Autodesk Inventor part; units mm, degrees
ref_plane "YZ Plane" through (0, 0, 0) normal (1, 0, 0) x (0, 1, 0)
ref_plane "XZ Plane" through (0, 0, 0) normal (0, 1, 0) x (-1, 0, 0)
ref_plane "XY Plane" through (0, 0, 0) normal (0, 0, 1) x (1, 0, 0)
sketch "Sketch1" plane through (0, 0, 0) normal (0, 1, 0) x (-1, 0, 0)
  circle A0 centre (-7.6905, 26.7159) radius 1.5
  circle A1 centre (-7.6905, 14.7159) radius 1.5
  line L0 (-0.1905, 5.7159) -> (-15.1905, 5.7159)
  line L1 (-15.1905, 35.7159) -> (-0.1905, 35.7159)
  line L2 (-15.1905, 5.7159) -> (-15.1905, 35.7159)
  circle A2 centre (5.6845, 41.7159) radius 1.5
  circle A3 centre (5.6845, 41.7159) radius 2.75
  line L3 (-2.528, 47.7159) -> (7.472, 47.7159)
  circle A4 centre (50.4345, -18.1591) radius 2.75
  circle A5 centre (50.4345, -36.2841) radius 1.5
  line L4 (9.8095, -42.2841) -> (9.8095, -22.2841)
  circle A6 centre (50.4345, -18.1591) radius 1.5
  line L5 (-0.1905, 35.7159) -> (-0.1905, 5.7159)
  line L6 (56.4345, 47.7159) -> (7.472, 47.7159)
  circle A7 centre (50.4345, 23.5909) radius 1.5
  line L7 (56.4345, -42.2841) -> (56.4345, 47.7159)
  line L8 (42.1595, 2.7159) -> (61.2095, 2.7159) construction
  circle A8 centre (50.4345, 23.5909) radius 2.75
  line L9 (-15.1905, 35.7159) -> (-30.1905, 35.7159)
  line L10 (-63.5655, 30.7159) -> (-63.5655, 47.7159)
  line L11 (-63.5655, 47.7159) -> (-48.5655, 47.7159)
  line L12 (-2.528, 47.7159) -> (-63.5655, 47.7159)
  circle A9 centre (-36.0655, 41.7159) radius 1.5
  circle A10 centre (-36.0655, 41.7159) radius 2.75
  circle A11 centre (-21.1905, -7.2841) radius 1.5
  line L13 (-27.6905, 2.7159) -> (-27.6905, -17.2841)
  circle A12 centre (-57.5655, -34.7841) radius 1.5
  line L14 (-2.6905, 2.7159) -> (-27.6905, 2.7159)
  circle A13 centre (-9.1905, -7.2841) radius 1.5
  line L15 (-2.6905, -17.2841) -> (-2.6905, 2.7159)
  line L16 (-27.6905, -17.2841) -> (-2.6905, -17.2841)
  line L17 (-63.5655, 47.7159) -> (-63.5655, -42.2841)
  line L18 (9.8095, -22.2841) -> (-40.1905, -22.2841)
  line L19 (-40.1905, -22.2841) -> (-40.1905, -42.2841)
  line L20 (-40.1905, -42.2841) -> (9.8095, -42.2841)
  line L21 (-63.5655, -42.2841) -> (56.4345, -42.2841)
  line L22 (-63.5655, 28.0659) -> (-48.5655, 28.0659)
  circle A14 centre (-22.6905, 26.7159) radius 1.5
  circle A15 centre (-53.0655, 20.5659) radius 1.5
  circle A16 centre (-59.0655, 20.5659) radius 1.5
  circle A17 centre (-53.0655, 20.5659) radius 2.5
  circle A18 centre (-22.6905, 14.7159) radius 1.5
  line L23 (-15.1905, 5.7159) -> (-15.1905, 35.7159)
  line L24 (-30.1905, 5.7159) -> (-15.1905, 5.7159)
  line L25 (-48.5655, 28.0659) -> (-48.5655, 13.0659)
  line L26 (-30.1905, 35.7159) -> (-30.1905, 5.7159)
  circle A19 centre (-59.0655, 20.5659) radius 2.5
  line L27 (-48.5655, 13.0659) -> (-63.5655, 13.0659)
  line L28 (-63.5655, 13.0659) -> (-63.5655, 28.0659)
  line L29 (-15.1905, 2.7159) -> (-15.1905, 34.925) construction
  line L30 (-48.5655, 28.0659) -> (-40.5655, 28.0659)
  line L31 (-40.5655, 28.0659) -> (-40.5655, 47.7159)
  point P0 (0, 0)
  point P1 (5.1035, 21.0043)
  point P2 (5.6845, 35.7159)
  point P3 (2.472, 2.7159)
  point P4 (-36.0655, 35.7159)
  point P5 (-2.6905, -7.2841)
  point P6 (-43.5655, 47.7159)
  dimension "d4" = 12
  dimension "d5" = 7.5
  dimension "d6" = 12
  dimension "d7" = 9
  dimension "d8" = 0
  dimension "d10" = 0
  dimension "d12" = 8
  dimension "d13" = 5.5
  dimension "d14" = 5.5
  dimension "d15" = 5.5
  dimension "d16" = 5.5
extrude "Extrusion1" add sketch "Sketch1" along normal blind 4 contours L3 L6 L7 L21 L4 L18 L19 L17 L27 L25 L30 L31 L12
extrude "Extrusion2" add sketch "Sketch1" along normal blind 2 contours L0 L2 L1 L5 | L24 L26 L9 L2 | A3 | L25 L27 L17 L22 | A4 | A8 | A10 | L14 L15 L16 L13 | A17 | A19
properties part number "Casis Kanan Bawah_3DPrint"
Build history of the part. All positions in model axes, mm. A direction names the side the tool comes from. Give positions to 0.01 mm unless a question says otherwise; leave off trailing zeros. Order: outer loops, then holes, each group sorted by start corner. A loop starts at its lowest first (then second) coordinate and runs counter-clockwise, first axis right, second up. Notation, with made-up numbers: M 50.25,-26 L 103.25,-26 A13 ccw 103.25,-5 Z; hole C 27.5,3.5 d1. An arc over 180 degrees is marked long. Put each result on its own line as item: value.
Item 1: Slice it at A-A, the plane z = -26. Write the cut outline in (x, y).
From the geometry:
outline: M -56.43,0 L -9.81,0 L -9.81,4 L -56.43,4 Z; M 40.19,0 L 63.57,0 L 63.57,4 L 40.19,4 Z
Item 2: Slice it at B-B, the plane z = 32. Write the cut outline in (x, y).
From the geometry:
outline: M -56.43,0 L 40.57,0 L 40.57,4 L 30.19,4 L 30.19,2 L 0.19,2 L 0.19,4 L -56.43,4 Z
Item 3: 3-axis set-ups, long thin cutter, end or side, ignore diameter. For faces 5 (the flat face through (15, 2, 21)), 6 (the flat face through (56, 2, 21)), 7 (the cylindrical face through (-51.127, 1.972, -34.953)): which of +Z, -Z, +X, -X, +Y, -Y reach the whole face in a straight line?
From the geometry:
face 5: +Y
face 6: +Z, +X, +Y
face 7: +Y, -Y
Item 4: Slice it at D-D, the plane x = 17.5. Write the cut outline in (y, z), plus the area to 3 significant figures.
From the geometry:
outline: M 0,-22.28 L 4,-22.28 L 4,-17.28 L 2,-17.28 L 2,2.72 L 4,2.72 L 4,5.72 L 2,5.72 L 2,35.72 L 4,35.72 L 4,47.72 L 0,47.72 Z
area: 180 mm2
Item 5: Probe line 1 (Z direction, x = 11, y = 3.1); line 2 (X direction, y = 3.85, z = -27); line 3 (Z direction, x = 21, y = 1.3). List the from-to ranges inside material, lowest first. Write a range as [from, to].
From the geometry:
line 1: z = [-22.28, -17.28], [2.72, 5.72], [35.72, 47.72]
line 2: x = [-56.43, -9.81], [40.19, 63.57]
line 3: z = [-22.28, -8.77], [-5.8, 47.72]
Item 6: Slice it at C-C, the plane y = 3.4. Give the number of separate pieces and of enclosed holes in the cut face, plus the area to 3 significant figures.
From the geometry:
separate pieces: 1
enclosed holes: 8
area: 7,610 mm2
Item 7: Flat gauge pins, fed straight in: pin 1 Ø6 at (x, z) = (37, 41) entering from +Y; pin 2 Ø2.5 at (x, z) = (-50.43, -18.16) entering from +Y; pin 3 Ø3.5 at (x, z) = (22.69, 26.72) entering from +Y; pin 4 Ø0.6 at (y, z) = (3, 24) entering from +X. Where does each tip first touch, or does it go through?
From the geometry:
pin 1: stops at y = 4
pin 2: passes through
pin 3: stops at y = 2
pin 4: stops at x = 48.57
Item 8: Two-plate mould, pull along Z, no slides. Class faces 1 (the flat face through (-56.434, 2, 2)), 2 (the flat face through (49.7, 1.5, 28.066)), 3 (the cylindrical face through (-51.241, 0.986, -19.424)), 4 (the cylindrical face through (-53.058, 2.986, 22.765)): +Z half, -Z half, draft (parallel to the pull), parting line (faces both ways), or undercut.
From the geometry:
face 1: draft
face 2: +Z half
face 3: undercut
face 4: undercut
